Here's how the part is built. I have some questions about the finished solid (model axes, mm). A direction names the side the tool comes from. Give positions to 0.01 mm unless a question says otherwise; leave off trailing zeros. Write each loop counter-clockwise with the first axis right and the second up, starting at its lowest first coordinate (ties: lowest second). Pieces come first, ordered by that corner, then holes. Notation, with made-up numbers: M 67,7 L 114,7 A5 cw 114,16 Z; hole C -24,35 d8. An arc over 180 degrees is marked long. Use one line per item in the form item = value. Start each with the question number.
from build123d import *

# Parameters (mm, degrees)
SKETCH_1_R      = 2
SKETCH_1_W      = 32
SKETCH_1_H      = 42.5
EXTRUDE_1_DEPTH = 3
SKETCH_2_W      = 38
SKETCH_2_H      = 8.5
EXTRUDE_2_DEPTH = 7
FILLET_1_R      = 1


with BuildPart() as part:
    # 草图1 → 凸台-拉伸1 (new body)
    with BuildSketch(Plane.XY):
        Polygon((0, 29.25), (23, 29.25), (23, -39.25), (-15, -39.25), (-15, 29.25), align=None)
        with Locations((4, 25.25)):
            Circle(SKETCH_1_R, mode=Mode.SUBTRACT)
        with Locations((4, -25.25)):
            Circle(SKETCH_1_R, mode=Mode.SUBTRACT)
        with Locations((4, 0)):
            Rectangle(SKETCH_1_W, SKETCH_1_H, mode=Mode.SUBTRACT)
    extrude(amount=EXTRUDE_1_DEPTH)

    # 草图2 → 凸台-拉伸2 (add)
    with BuildSketch(Plane(origin=(0, 0, 0), x_dir=(-1, 0, 0), z_dir=(0, 0, -1))):
        with Locations((-4, -35)):
            Rectangle(SKETCH_2_W, SKETCH_2_H)
    extrude(amount=EXTRUDE_2_DEPTH)

    # 圆角1
    fillet_1_edges = [part.edges().sort_by_distance(p)[0] for p in [
        (-12, -21.25, 1.5),
        (20, -21.25, 1.5),
        (20, 21.25, 1.5),
        (-12, 21.25, 1.5),
        (23, -0.75, 0),
        (23, -30.75, -3.5),
        (4, -30.75, 0),
        (-15, -30.75, -3.5),
        (-15, -0.75, 0),
        (-15, -39.25, -2),
        (-15, 29.25, 1.5),
        (23, 29.25, 1.5),
        (23, -39.25, -2),
    ]]
    fillet(fillet_1_edges, radius=FILLET_1_R)


solid = part.part
1) Suppose I cut it at A-A, the plane y = -25.25. List the corners of the cut face in (x, z) for me, and give its area (3 significant figures).
2) Suppose I cut it at D-D, the plane x = 15.5. List the corners of the cut face in (y, z) for me, and give its area (3 significant figures).
3) Suppose I cut it at B-B, the plane x = 4. List the corners of the cut face in (y, z) for me, and give its area (3 significant figures).
4) Please list where these lines run through material, in increasing order: line 1 (Y direction, x = 4, z = 2.35); line 2 (X direction, y = 19, z = 2.25); line 3 (Y direction, x = 13.5, z = 2.5).
5) On a 3-axis mill with a long thin cutter (end or side, diameter ignored), from which of +Z, -Z, +X, -X, +Y, -Y can I reach the whole of each face in a straight line? I mean faces 5 (the face through (21, 2, 0)), 6 (the face through (-12, 0, 1)), 7 (the face through (4, -35, -7)). Say none if no direction works.
6) Will these pins go through, and if not, where does the flat tip stop? P1, Ø3, axis at x = 19, z = -3, coming from the +Y side; P2, Ø6.5, axis at x = 4, y = -25.25, coming from the -Z side.
7) Suppose I cut it at C-C, the plane z = -2. List the corners of the cut face in (x, y) for me, and give its area (3 significant figures).
8) Thinking about a two-plate mould opening in Y: for faces 1 (the face through (4, -21.25, 1)), 2 (the face through (4, 29.25, 1)), 3 (the face through (4, -39.25, -2)), 4 (the face through (23, -15, 2)), which applies, released by +Y, released by -Y, zero draft, split by the parting line, or undercut?
Checks:
q1.outline = M -15,1 A1 ccw -14,0 L 2,0 L 2,3 L -15,3 Z; M 6,0 L 22,0 A1 ccw 23,1 L 23,3 L 6,3 Z
q1.area = 102 mm^2
q2.outline = M -39.25,-7 L -30.75,-7 L -30.75,-1 A1 cw -29.75,0 L -21.25,0 L -21.25,3 L -39.25,3 Z; M 21.25,0 L 29.25,0 L 29.25,3 L 21.25,3 Z
q2.area = 138 mm^2
q3.outline = M -39.25,-7 L -30.75,-7 L -30.75,-1 A1 cw -29.75,0 L -27.25,0 L -27.25,3 L -39.25,3 Z; M -23.25,0 L -21.25,0 L -21.25,3 L -23.25,3 Z; M 21.25,0 L 23.25,0 L 23.25,3 L 21.25,3 Z; M 27.25,0 L 29.25,0 L 29.25,3 L 27.25,3 Z
q3.area = 114 mm^2
q4.line_1 = -39.25 to -27.25, -23.25 to -21.25, 21.25 to 23.25, 27.25 to 29.25
q4.line_2 = -15 to -12, 20 to 23
q4.line_3 = -39.25 to -21.25, 21.25 to 29.25
q5.face_5 = -Z, +X, -X, +Y
q5.face_6 = +Z, -Z
q5.face_7 = -Z, +X, -X, +Y, -Y
q6.P1 = -30.75
q6.P2 = 0
q7.outline = M -15,-38.25 A1 ccw -14,-39.25 L 22,-39.25 A1 ccw 23,-38.25 L 23,-31.75 A1 ccw 22,-30.75 L -14,-30.75 A1 ccw -15,-31.75 Z
q7.area = 322 mm^2
q8.face_1 = undercut
q8.face_2 = released by +Y
q8.face_3 = released by -Y
q8.face_4 = zero draft
